Source: CAD feature listing. Evaluate the final solid. Frame: model axes, mm. A direction names the side the tool comes from. Coordinates: 2 decimals unless noted, no trailing zeros. Order: outer loops, then holes, each group sorted by start corner. A loop starts at its lowest first (then second) coordinate and runs counter-clockwise, first axis right, second up.
```python
from build123d import *


with BuildPart() as part:
    # Croquis1 → Revolución1 (revolve)
    with BuildSketch(Plane.XY):
        Polygon((0, 50), (8, 50), (8, 17.5), (6, 17.5), (6, 15.5), (8, 15.5), (8, 14), (6, 14), (6, 12), (8, 12), (8, 10.5), (6, 10.5), (6, 8.5), (8, 8.5), (8, 7), (6, 7), (6, 5), (8, 5), (8, 3.5), (6, 3.5), (6, 1.5), (8, 1.5), (8, 0), (4, 0), (4, -2), (0, -2), (0, 0), align=None)
    revolve(axis=Axis((0, 68.764044944, 0), (0, -1, 0)))


solid = part.part
```
Q1. Pin query (flat end, axial travel): P1, Ø1.5, axis at y = 17, z = 1, coming from the +X side; P2, Ø4, axis at x = 3, y = 26.5, coming from the -Z side. Return the tip coordinate at first contact, or that it passes through.
Solutions:
P1: stops at x = 7.99
P2: stops at z = -7.94
Q2. Set-up query: faces 4 (the cylindrical face through (-1.73, 14.74, -7.81)), 5 (the cylindrical face through (-0.867, -1.014, -3.905)), 6 (the flat face through (-2, 17.5, 6)). Return all of +Z, -Z, +X, -X, +Y, -Y with unobstructed straight access to the full face (end or side cutting, diameter ignored); none if empty.
Solutions:
face 4: +Y, -Y
face 5: -Y
face 6: none
Q3. Material intervals for line 1 along Y through (x, z) = (2.5, 7.25); line 2 along Y through (x, z) = (-0.5, 5.25); line 3 along Z through (x, y) = (5.25, 9), sorted ascending.
Solutions:
line 1: y = 0 to 1.5, 3.5 to 5, 7 to 8.5, 10.5 to 12, 14 to 15.5, 17.5 to 50
line 2: y = 0 to 50
line 3: z = -2.9 to 2.9
Q4. Pull-direction query (Y, two-part tool) for faces 1 (the flat face through (2, 12, 6)), 2 (the flat face through (-4, 0, -2)), 3 (the cylindrical face through (-1.73, 0.74, -7.81)); classes: pulls with the +Y half, pulls with the -Y half, needs draft (parallel to the pull), parting line crosses it, or undercut.
Solutions:
face 1: undercut
face 2: pulls with the -Y half
face 3: needs draft
Q5. Section query B-B on y = 18. Output: boundary loops of the cut face in (x, z), plus the area to 3 significant figures.
Solutions:
outline: circle Ø16 at (0, 0)
area: 201 mm2
Q6. Section query A-A on z = 6.75. Output: boundary loops of the cut face in (x, y).
Solutions:
outline: (-4.29, 0) - (4.29, 0) - (4.29, 1.5) - (-4.29, 1.5) - close; (-4.29, 3.5) - (4.29, 3.5) - (4.29, 5) - (-4.29, 5) - close; (-4.29, 7) - (4.29, 7) - (4.29, 8.5) - (-4.29, 8.5) - close; (-4.29, 10.5) - (4.29, 10.5) - (4.29, 12) - (-4.29, 12) - close; (-4.29, 14) - (4.29, 14) - (4.29, 15.5) - (-4.29, 15.5) - close; (-4.29, 17.5) - (4.29, 17.5) - (4.29, 50) - (-4.29, 50) - close
